from build123d import *

# Parameters (mm, degrees)
F0_W      = 14.75
F0_H      = 14.75
F0_W_2    = 10.25
F0_H_2    = 10.25
F1_DEPTH  = 14.5200116
F2_W      = 14.75
F2_H      = 14.75
F2_W_2    = 10.25
F2_H_2    = 10.25
F3_DEPTH  = 14.5200116
F4_W      = 14.75
F4_H      = 14.5200116
F5_DEPTH  = 14.5200116
F6_W      = 14.75
F6_H      = 14.5200116
F6_W_2    = 10.25
F6_H_2    = 10.25
F7_DEPTH  = 14.5200116
F8_R      = 1.6
F9_DEPTH  = 25.4
F10_R     = 1.6
F11_DEPTH = 25.4
F12_R     = 1.6
F13_DEPTH = 25.4
F14_R     = 1.6
F15_DEPTH = 25.4


with BuildPart() as f1:
    # F0 (on Top) → F1 (new body)
    with BuildSketch(Plane.XY):
        with Locations((5.125, -5.125)):
            Rectangle(F0_W, F0_H)
        with Locations((5.125, -5.125)):
            Rectangle(F0_W_2, F0_H_2, mode=Mode.SUBTRACT)
    extrude(amount=F1_DEPTH)

    # F2 (on face) → F3 (join)
    with BuildSketch(Plane(origin=(0, 0, 0), x_dir=(1, 0, 0), z_dir=(0, 0, -1))):
        with Locations((5.125, 5.125)):
            Rectangle(F2_W, F2_H)
        with Locations((5.125, 5.125)):
            Rectangle(F2_W_2, F2_H_2, mode=Mode.SUBTRACT)
        with Locations((5.125, 5.125)):
            Rectangle(F2_W_2, F2_H_2)
    extrude(amount=F3_DEPTH)

    # F4 (on face) → F5 (join)
    with BuildSketch(Plane.XZ.offset(12.5)):
        with Locations((5.125, -7.2600058)):
            Rectangle(F4_W, F4_H)
        Polygon((0, -12.2700116), (0, -2.25), (10.25, -2.25), (10.25, -12.2700116), (10.25, -12.5), (0, -12.5), align=None, mode=Mode.SUBTRACT)
    extrude(amount=F5_DEPTH)

    # F6 (on face) → F7 (join)
    with BuildSketch(Plane.YZ.offset(12.5)):
        with Locations((-5.125, -7.2600058)):
            Rectangle(F6_W, F6_H)
        with Locations((-5.125, -7.1450116)):
            Rectangle(F6_W_2, F6_H_2, mode=Mode.SUBTRACT)
    extrude(amount=F7_DEPTH)

    # F8 (on face) → F9 (cut)
    with BuildSketch(Plane.XZ.offset(12.5)):
        with Locations((17.25, -7.2600058)):
            Circle(F8_R)
    extrude(amount=-F9_DEPTH, mode=Mode.SUBTRACT)

    # F10 (on face) → F11 (cut)
    with BuildSketch(Plane.YZ.offset(12.5)):
        with Locations((-17.25, -7.2600058)):
            Circle(F10_R)
    extrude(amount=-F11_DEPTH, mode=Mode.SUBTRACT)

    # F12 (on face) → F13 (cut)
    with BuildSketch(Plane(origin=(-2.25, 0, 0), x_dir=(0, -1, 0), z_dir=(-1, 0, 0))):
        with Locations((5.125, 4.75)):
            Circle(F12_R)
    extrude(amount=-F13_DEPTH, mode=Mode.SUBTRACT)

    # F14 (on face) → F15 (cut)
    with BuildSketch(Plane.XZ.offset(12.5)):
        with Locations((5.125, 4.75)):
            Circle(F14_R)
    extrude(amount=-F15_DEPTH, mode=Mode.SUBTRACT)


solid = f1.part
Can you work these out from the model? Positions are in its coordinate system, mm. A direction names the side the tool comes from. Round coordinates to 2 decimals unless told otherwise and drop trailing zeros. Write each loop counter-clockwise with the first axis right and the second up, starting at its lowest first coordinate (ties: lowest second). Pieces come first, ordered by that corner, then holes. Notation, with made-up numbers: (7, -9) -> (50, -9) arc R27 ccw to (50, 18) -> close; hole circle Ø5 at (39.5, 24.25). An arc over 180 degrees is marked (long way). One line per question, with ' | ' between items. Start each with the question number.
1) Suppose I cut it at B-B on z = 4.75. Write out the boundary of the cut face in (x, y) (3 decimals).
2) On a 3-axis mill with a long thin cutter (end or side, diameter ignored), from which of +Z, -Z, +X, -X, +Y, -Y can I reach the whole of each face in a straight line? I mean faces 1 (the flat face through (5, -12.5, 7)), 2 (the flat face through (20, -5, -12.27)), 3 (the flat face through (5, -12.5, -7)), 4 (the flat face through (5, -10.25, 7)), 5 (the cylindrical face through (-1.11, -18.43, -6.18)). Say none if no direction works.
3) Suppose I cut it at C-C on z = 1.75. Write out the boundary of the cut face in (x, y).
4) If we mould it in two halves opening along Z, with no side actions, what happens to faces 6 (the flat face through (5, 0, 7)), 7 (the flat face through (-2, -5, 14.52)), 8 (the flat face through (20, -10.25, -7))? For each: released by +Z, released by -Z, zero draft, split by the parting line, or undercut.
5) I need wall thicknesses on line 1 (Z direction, x = 14.25, y = -1.5); line 2 (Y direction, x = 10, z = 8.75); line 3 (Z direction, x = 11, y = -17.25). Which ranges of each line are inside material? Lowest first, please. Write a range as [from, to].
6) Suppose I cut it at A-A on x = 17.25. Write out the boundary of the cut face in (y, z), then the cut area to 3 significant figures.
7) Suppose I cut it at D-D on y = -17.25. Write out the boundary of the cut face in (x, z), then the cut area to 3 significant figures.
8) I'm going to push flat-ended pins straight in: P1, Ø3, axis at y = -23.5, z = -0.5, coming from the +X side; P2, Ø11.5, axis at x = 5, y = -21, coming from the +Z side; P3, Ø5, axis at x = 5.5, z = -9, coming from the -Y side. Where does each tip first touch, or does it pass through?
Return value:
1) outline: (-2.25, -12.5) -> (3.525, -12.5) -> (3.525, -10.25) -> (0, -10.25) -> (0, -6.725) -> (-2.25, -6.725) -> close; (-2.25, -3.525) -> (0, -3.525) -> (0, 0) -> (3.525, 0) -> (3.525, 2.25) -> (-2.25, 2.25) -> close; (6.725, -12.5) -> (12.5, -12.5) -> (12.5, -6.725) -> (10.25, -6.725) -> (10.25, -10.25) -> (6.725, -10.25) -> close; (6.725, 0) -> (10.25, 0) -> (10.25, -3.525) -> (12.5, -3.525) -> (12.5, 2.25) -> (6.725, 2.25) -> close
2) face 1: +Z, +X, -X, -Y | face 2: +X | face 3: -Y | face 4: +Z | face 5: +X, -X
3) outline: (-2.25, -12.5) -> (12.5, -12.5) -> (12.5, 2.25) -> (-2.25, 2.25) -> close; hole (0, -10.25) -> (10.25, -10.25) -> (10.25, 0) -> (0, 0) -> close
4) face 6: zero draft | face 7: released by +Z | face 8: undercut
5) line 1: z = [-14.52, -12.27], [-2.02, 0] | line 2: y = [-12.5, -10.25], [0, 2.25] | line 3: z = [-14.52, -8.86], [-5.66, 0]
6) outline: (-12.5, -14.52) -> (2.25, -14.52) -> (2.25, -8.86) -> (0, -8.86) -> (0, -12.27) -> (-10.25, -12.27) -> (-10.25, -8.86) -> (-12.5, -8.86) -> close; (-12.5, -5.66) -> (-10.25, -5.66) -> (-10.25, -2.02) -> (0, -2.02) -> (0, -5.66) -> (2.25, -5.66) -> (2.25, 0) -> (-12.5, 0) -> close | area: 94.7 mm2
7) outline: (-2.25, -14.52) -> (12.5, -14.52) -> (12.5, -8.86) -> (10.25, -8.86) -> (10.25, -12.5) -> (0, -12.5) -> (0, -8.86) -> (-2.25, -8.86) -> close; (-2.25, -5.66) -> (0, -5.66) -> (0, -2.25) -> (10.25, -2.25) -> (10.25, -5.66) -> (12.5, -5.66) -> (12.5, 0) -> (-2.25, 0) -> close | area: 94.7 mm2
8) P1: stops at x = 12.5 | P2: stops at z = 0 | P3: stops at y = -12.5
